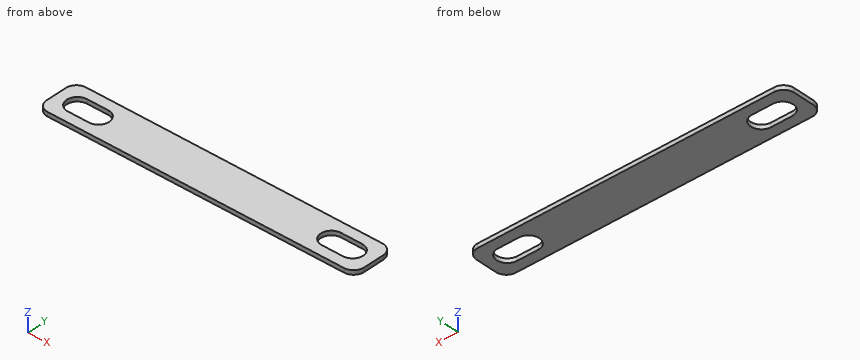
```python
from build123d import *

# Parameters (mm, degrees)
SKETCH074_W     = 2
SKETCH074_H     = 0.2
PAD047_DEPTH    = 7.5
POCKET021_DEPTH = 0.2
FILLET019_R     = 0.5


with BuildPart() as part:
    # Sketch074 → Pad047 (new body, symmetric)
    with BuildSketch(Plane.YZ):
        with Locations((21.35, -8.25)):
            Rectangle(SKETCH074_W, SKETCH074_H)
    extrude(amount=PAD047_DEPTH, both=True)

    # Sketch075 (on Face3 of Pad047) → Pocket021 (cut)
    with BuildSketch(Plane.YX.offset(8.35)):
        with BuildLine():
            ThreePointArc((21.85, 6.4999958532), (21.35, 7), (20.85, 6.4999958531))
            Line((20.85, 6.4999958531), (20.85, 5.4999999932))
            ThreePointArc((20.85, 5.4999999932), (21.35, 5), (21.85, 5.4999999932))
            Line((21.85, 6.4999958532), (21.85, 5.4999999932))
        make_face()
        with BuildLine():
            ThreePointArc((20.85, -6.4999958531), (21.35, -7), (21.85, -6.4999958532))
            Line((21.85, -6.4999958532), (21.85, -5.4999999932))
            ThreePointArc((21.85, -5.4999999932), (21.35, -5), (20.85, -5.4999999932))
            Line((20.85, -6.4999958531), (20.85, -5.4999999932))
        make_face()
    extrude(amount=-POCKET021_DEPTH, mode=Mode.SUBTRACT)

    # Fillet019
    fillet019_edges = [part.edges().sort_by_distance(p)[0] for p in [
        (-7.5, 22.35, -8.25),
        (-7.5, 20.35, -8.25),
        (7.5, 20.35, -8.25),
        (7.5, 22.35, -8.25),
    ]]
    fillet(fillet019_edges, radius=FILLET019_R)


with BuildPart() as part_1:
    # Body026 placement: moved
    add(part.part.moved(Location((0, 25.7, 0))))


solid = part_1.part
```
Model file for the job. Use its own axes, mm. Coordinates: 2 decimals unless noted, no trailing zeros. Loops run counter-clockwise (first coordinate to the right, second up) from the corner with the lowest first, then second, coordinate; pieces in that order, holes last. Notation, with made-up numbers: (83.5, -15.75) - (104.5, -15.75) arc R25 ccw to (104.5, 6.25) - close; hole circle Ø7 at (74.25, 45.25). An arc over 180 degrees is marked (long way). Answer as a JSON object with one key per item and string values. Group by question number.
(1) Cut at A-A (y = 47.05). Give the cut face in (x, z).
(2) Cut at B-B (z = -8.2). Give the cut face in (x, y), then the cut area to 3 significant figures.
(3) Probe line 1 along X through (y, z) = (47.05, -8.3); line 2 along Y through (x, z) = (5.5, -8.2); line 3 along X through (y, z) = (47.3, -8.2). List the from-to ranges inside material, lowest first.
Geometry says:
{
 "1": {"outline": "(-7.5, -8.35) - (-7, -8.35) - (-7, -8.15) - (-7.5, -8.15) - close; (-5, -8.35) - (5, -8.35) - (5, -8.15) - (-5, -8.15) - close; (7, -8.35) - (7.5, -8.35) - (7.5, -8.15) - (7, -8.15) - close"},
 "2": {"outline": "(-7.5, 46.55) arc R0.5 ccw to (-7, 46.05) - (7, 46.05) arc R0.5 ccw to (7.5, 46.55) - (7.5, 47.55) arc R0.5 ccw to (7, 48.05) - (-7, 48.05) arc R0.5 ccw to (-7.5, 47.55) - close; hole (-6.5, 46.55) - (-5.5, 46.55) arc R0.5 ccw to (-5.5, 47.55) - (-6.5, 47.55) arc R0.5 ccw to start; hole (5.5, 46.55) - (6.5, 46.55) arc R0.5 ccw to (6.5, 47.55) - (5.5, 47.55) arc R0.5 ccw to start", "area": "26.2 mm^2"},
 "3": {"line 1": "x = -7.5 to -7, -5 to 5, 7 to 7.5", "line 2": "y = 46.05 to 46.55, 47.55 to 48.05", "line 3": "x = -7.5 to -6.93, -5.07 to 5.07, 6.93 to 7.5"}
}
